Part model, mm, in its own coordinate system. Face numbers are marked on the shaded views. Coordinates: 2 decimals unless noted, no trailing zeros. Order: outer loops, then holes, each group sorted by start corner. A loop starts at its lowest first (then second) coordinate and runs counter-clockwise, first axis right, second up.
from build123d import *

# Parameters (mm, degrees)
SKETCH1_R                = 2.5
BOSS_EXTRUDE1_DEPTH      = 13
F_2_0_2_DIAMETER_HOLE1_D = 2
CHAMFER2_SIZE            = 1


with BuildPart() as part:
    # Sketch1 → Boss-Extrude1 (new body)
    with BuildSketch(Plane.XY):
        Circle(SKETCH1_R)
    extrude(amount=BOSS_EXTRUDE1_DEPTH)

    # Sketch3 → Cut-Revolve1 (revolve, cut)
    with BuildSketch(Plane(origin=(0, 0, 0), x_dir=(1, 0, 0), z_dir=(0, 1, 0))):
        with BuildLine():
            Line((3.138230266, -4), (2.2, -4))
            ThreePointArc((2.2, -4), (1.634314575, -4.234314575), (1.4, -4.8))
            Line((1.4, -4.8), (1.4, -7.2))
            ThreePointArc((1.4, -7.2), (1.634314575, -7.765685425), (2.2, -8))
            Line((2.2, -8), (3.138230266, -8))
            Line((3.138230266, -8), (3.138230266, -4))
        make_face()
    revolve(axis=Axis((0, 0, 0), (0, 0, 1)), mode=Mode.SUBTRACT)

    # Ø2.0 (2) Diameter Hole1 (through all)
    with Locations(Plane.XY.offset(13)):
        with Locations((0, 0)):
            Hole(F_2_0_2_DIAMETER_HOLE1_D / 2)

    # Chamfer2
    chamfer2_edges = [part.edges().sort_by_distance(p)[0] for p in [
        (1, 0, 13),
    ]]
    chamfer(chamfer2_edges, length=CHAMFER2_SIZE)


solid = part.part
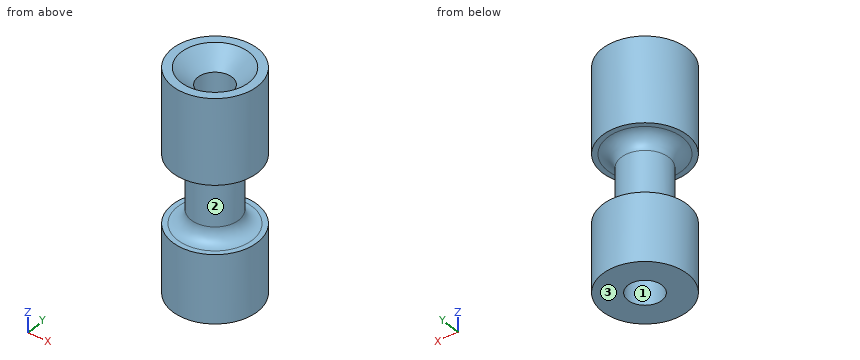
Q1. Mould opens along X. For the marked faces 1, 2 and 3 say: pulls with the +X half, pulls with the -X half, needs draft (parallel to the pull), parting line crosses it, or undercut.
Results list:
face 1: undercut
face 2: parting line crosses it
face 3: needs draft
Q2. Cut at A-A on y = 0. Write the cut outline in (x, z), and give its area (3 significant figures).
Results list:
outline: (-2.5, 0) - (-1, 0) - (-1, 12) - (-2, 13) - (-2.5, 13) - (-2.5, 8) - (-2.2, 8) arc R0.8 cw to (-1.4, 7.2) - (-1.4, 4.8) arc R0.8 cw to (-2.2, 4) - (-2.5, 4) - close; (1, 0) - (2.5, 0) - (2.5, 4) - (2.2, 4) arc R0.8 cw to (1.4, 4.8) - (1.4, 7.2) arc R0.8 cw to (2.2, 8) - (2.5, 8) - (2.5, 13) - (2, 13) - (1, 12) - close
area: 29.7 mm2
Q3. Cut at D-D on z = 1.5. Write the cut outline in (x, y).
Results list:
outline: circle Ø5 at (0, 0); hole circle Ø2 at (0, 0)
Q4. Wall check: line 1 along Z through (x, y) = (1.65, 1.55); line 2 along Y through (x, z) = (0, 4.75); line 3 along Y through (x, z) = (0, 9.25). Give the ranges that are in metal, low to high.
Results list:
line 1: z = 0 to 4, 8 to 13
line 2: y = -1.4 to -1, 1 to 1.4
line 3: y = -2.5 to -1, 1 to 2.5
Q5. Cut at C-C on z = 5.5. Write the cut outline in (x, y).
Results list:
outline: circle Ø2.8 at (0, 0); hole circle Ø2 at (0, 0)
Q6. Pin check, flat tip, straight feed: pin 1 Ø1.5 at (x, y) = (0, 1) entering from +Z. Stop position of the tip, or through.
Results list:
pin 1: stops at z = 12.75
